```python
from build123d import *

# Parameters (mm, degrees)
F0_W     = 2.54
F0_H     = 3.81
F0_W_2   = 3.81
F0_H_2   = 73.66
F1_DEPTH = 3.175
F2_DEPTH = 9.7028
F3_START = 6.35
F3_DEPTH = 3.3528


with BuildPart() as f1:
    # F0 (on Top) → F1 (new body)
    with BuildSketch(Plane.XY):
        Polygon((-55.88, -36.83), (-55.88, 36.83), (55.88, 36.83), (59.69, 36.83), (59.69, 40.64), (-59.69, 40.64), (-59.69, -40.64), (59.69, -40.64), (59.69, -36.83), (55.88, -36.83), align=None)
        with Locations((60.96, 38.735)):
            Rectangle(F0_W, F0_H)
        with Locations((60.96, -38.735)):
            Rectangle(F0_W, F0_H)
        with Locations((57.785, 0)):
            Rectangle(F0_W_2, F0_H_2)
        with Locations((60.96, 0)):
            Rectangle(F0_W, F0_H_2)
    extrude(amount=F1_DEPTH)

    # F0 (on Top) → F2 (join)
    with BuildSketch(Plane.XY):
        Polygon((-59.69, 40.64), (59.69, 40.64), (62.23, 40.64), (62.23, 43.18), (-62.23, 43.18), (-62.23, -43.18), (62.23, -43.18), (62.23, -40.64), (59.69, -40.64), (-59.69, -40.64), align=None)
    extrude(amount=F2_DEPTH)

    # F0 (on Top) → F3 (join)
    with BuildSketch(Plane.XY.offset(F3_START)):
        Polygon((-55.88, -36.83), (-55.88, 36.83), (55.88, 36.83), (59.69, 36.83), (59.69, 40.64), (-59.69, 40.64), (-59.69, -40.64), (59.69, -40.64), (59.69, -36.83), (55.88, -36.83), align=None)
        with Locations((60.96, -38.735)):
            Rectangle(F0_W, F0_H)
        with Locations((60.96, 38.735)):
            Rectangle(F0_W, F0_H)
    extrude(amount=F3_DEPTH)


solid = f1.part
```
Design review of the part built by this model. Coordinates are the model's own, in mm. A direction names the side the tool comes from. Coordinates: 2 decimals unless noted, no trailing zeros. Loops run counter-clockwise (first coordinate to the right, second up) from the corner with the lowest first, then second, coordinate; pieces in that order, holes last. Notation, with made-up numbers: (-18, 35.25) -> (22, 35.25) arc R28 cw to (22, 70.25) -> close; hole circle Ø7 at (-7.5, 48.25). An arc over 180 degrees is marked (long way). Answer as a JSON object with one key per item and string values.
Q1. Tool access review of faces 1 (the flat face through (55.88, -1, 2)), 2 (the flat face through (-5, -38, 0)), 3 (the flat face through (-17, -39, 6.35)), 4 (the flat face through (-55.88, -1, 8)): name each direction out of +Z, -Z, +X, -X, +Y, -Y from which nothing blocks a thin tool from reaching the whole face with its end or side.
Answer block:
{"face 1": "+Z, -Z", "face 2": "-Z, +X, -X, +Y, -Y", "face 3": "+X", "face 4": "+Z, -Z, +X"}
Q2. Clearance check with flat-ended pins moving along their axes: pin 1 Ø1.6 at (y, z) = (-4.5, 5) entering from +X; pin 2 Ø3.5 at (y, z) = (-13, 7.5) entering from +X. State where each tip first meets the part, or that it passes through.
Answer block:
{"pin 1": "stops at x = -59.69", "pin 2": "stops at x = -55.88"}
Q3. Take a section at C-C on z = 1.75. Give the boundary of the cut face in (x, y), plus the area to 3 significant figures.
Answer block:
{"outline": "(-62.23, -43.18) -> (62.23, -43.18) -> (62.23, 43.18) -> (-62.23, 43.18) -> close; hole (-55.88, -36.83) -> (55.88, -36.83) -> (55.88, 36.83) -> (-55.88, 36.83) -> close", "area": "2,520 mm^2"}
Q4. The part is to be moulded in two halves that separate along Z. For faces 5 (the flat face through (-10, -38, 9.703)), 6 (the flat face through (-59.69, -1, 5)), 7 (the flat face through (62.23, -1, 3)), say which applies: +Z half, -Z half, draft (parallel to the pull), parting line (faces both ways), or undercut.
Answer block:
{"face 5": "+Z half", "face 6": "undercut", "face 7": "draft"}
Q5. To check wall thickness, follow L1, parallel to Y at x = 40.5, z = 1; L2, parallel to Y at x = 7, z = 6; L3, parallel to X at y = 11.5, z = 2.75. State the ranges of each line that lie inside material, in increasing order.
Answer block:
{"L1": "y = -43.18 to -36.83, 36.83 to 43.18", "L2": "y = -43.18 to -40.64, 40.64 to 43.18", "L3": "x = -62.23 to -55.88, 55.88 to 62.23"}
Q6. Take a section at B-B on y = -8.5. Give the boundary of the cut face in (x, z) (3 decimals), plus the area to 3 significant figures.
Answer block:
{"outline": "(-62.23, 0) -> (-55.88, 0) -> (-55.88, 3.175) -> (-59.69, 3.175) -> (-59.69, 6.35) -> (-55.88, 6.35) -> (-55.88, 9.703) -> (-62.23, 9.703) -> close; (55.88, 0) -> (62.23, 0) -> (62.23, 3.175) -> (55.88, 3.175) -> close", "area": "69.7 mm^2"}
Q7. Take a section at A-A on x = 25. Give the boundary of the cut face in (y, z) (3 decimals), plus the area to 3 significant figures.
Answer block:
{"outline": "(-43.18, 0) -> (-36.83, 0) -> (-36.83, 3.175) -> (-40.64, 3.175) -> (-40.64, 6.35) -> (-36.83, 6.35) -> (-36.83, 9.703) -> (-43.18, 9.703) -> close; (36.83, 0) -> (43.18, 0) -> (43.18, 9.703) -> (36.83, 9.703) -> (36.83, 6.35) -> (40.64, 6.35) -> (40.64, 3.175) -> (36.83, 3.175) -> close", "area": "99.0 mm^2"}
